Autodesk Fusion 360 part; units mm, degrees
sketch "Sketch1" plane through (0, 0, 0) normal (1, 0, 0) x (0, 1, 0)
  line L0 (180, 75) -> (-180, 75)
  line L1 (-240, 15) -> (-240, -75)
  line L2 (240, -75) -> (240, 15)
  line L3 (-240, -75) -> (-180, -75)
  line L4 (-180, -75) -> (-180, 75)
  line L5 (-240, 15) -> (-240, -75)
  line L6 (240, -75) -> (180, -75)
  line L7 (180, -75) -> (180, 75)
  line L8 (240, 15) -> (240, -75)
  line L9 (-180, 75) -> (180, 75)
  line L10 (240, 15) -> (-240, 15)
  line L11 (-240, 15) -> (-180, 75)
  line L12 (240, 15) -> (180, 75)
  line L13 (-240, -75) -> (-180, -75)
  line L14 (180, -75) -> (240, -75)
  line L15 (194.2857, 60.7143) -> (48, 15) construction
  line L16 (-194.2857, 60.7143) -> (-48, 15) construction
  line L17 (180, -56.25) -> (240, -75) construction
  line L18 (0, 55) -> (5, 55)
  line L19 (5, 35) -> (0, 35)
  line L20 (5, 65) -> (10, 65)
  line L21 (10, 65) -> (10, 25)
  line L22 (10, 25) -> (5, 25)
  line L23 (0, 75) -> (0, 55)
  line L24 (0, 35) -> (0, 15)
  line L25 (5, 25) -> (5, 35)
  line L26 (5, 55) -> (5, 65)
  dimension "d1" = 480
  dimension "d3" = 60
  dimension "d5" = 60
extrude "Extrude1" add sketch "Sketch1" along normal blind 3
sketch "Sketch2" plane through (0, 0, 0) normal (-1, 0, 0) x (0, -1, 0)
  line L0 (-180, -75) -> (-180, 15)
  line L1 (-180, 15) -> (180, 15)
  line L2 (180, 15) -> (180, -75)
  line L3 (180, -75) -> (240, -75)
  line L4 (240, -75) -> (240, 15)
  line L5 (240, 15) -> (180, 75)
  line L6 (180, 75) -> (-180, 75)
  line L7 (-180, 75) -> (-240, 15)
  line L8 (-240, 15) -> (-240, -75)
  line L9 (-240, -75) -> (-180, -75)
  line L10 (0, 55) -> (5, 55)
  line L11 (5, 35) -> (0, 35)
  line L12 (5, 65) -> (10, 65)
  line L13 (10, 65) -> (10, 25)
  line L14 (10, 25) -> (5, 25)
  line L15 (5, 25) -> (5, 35)
  line L16 (5, 55) -> (5, 65)
  line L17 (0, 55) -> (0, 75)
  line L18 (0, 35) -> (0, 15)
fillet "Fillet1" radius 25 2 edges at (1.5, -180, 15) (1.5, 180, 15)
fillet "Fillet2" radius 25 4 edges at (1.5, -240, 15) (1.5, -180, 75) (1.5, 180, 75) (1.5, 240, 15)
sketch "Sketch3" plane through (3, 0, 0) normal (1, 0, 0) x (0, 1, 0)
  arc A0 (240, 4.6447) -> (232.6777, 22.3223) centre (215, 4.6447) ccw
  line L0 (232.6777, 22.3223) -> (187.3223, 67.6777)
  arc A1 (187.3223, 67.6777) -> (169.6447, 75) centre (169.6447, 50) ccw
  line L1 (169.6447, 75) -> (-169.6447, 75)
  arc A2 (-169.6447, 75) -> (-187.3223, 67.6777) centre (-169.6447, 50) ccw
  line L2 (-187.3223, 67.6777) -> (-232.6777, 22.3223)
  arc A3 (-232.6777, 22.3223) -> (-240, 4.6447) centre (-215, 4.6447) ccw
  line L3 (-240, 4.6447) -> (-240, -75)
  line L4 (-240, -75) -> (-180, -75)
  line L5 (-180, -75) -> (-180, -10)
  arc A4 (-155, 15) -> (-180, -10) centre (-155, -10) ccw
  line L6 (-155, 15) -> (155, 15)
  arc A5 (180, -10) -> (155, 15) centre (155, -10) ccw
  line L7 (180, -10) -> (180, -75)
  line L8 (180, -75) -> (240, -75)
  line L9 (240, -75) -> (240, 4.6447)
The listing builds one solid part. Answer for the finished solid, in the listing's coordinates (mm). A direction names the side the tool comes from. Give positions to 0.01 mm unless a question says otherwise; leave off trailing zeros. Write each loop counter-clockwise with the first axis right and the second up, starting at its lowest first coordinate (ties: lowest second). Pieces come first, ordered by that corner, then holes.
Item 1: Which of the six approach directions +Z, -Z, +X, -X, +Y, -Y give full straight-line access (tool end or side, diameter ignored) to faces 1 (the cylindrical face through (1.521, 172.871, 7.482)), 2 (the flat face through (1, 210, 45))?
Item 2: Section C-C, the plane y = 67 is taken. Write down the section's boundary in (x, z), plus the area to 3 significant figures.
Item 3: Section A-A, the plane z = -25 is taken. Write down the section's boundary in (x, y), plus the area to 3 significant figures.
Item 4: Section D-D, the plane y = -161.5 is taken. Write down the section's boundary in (x, z), plus the area to 3 significant figures.
Item 5: Section B-B, the plane x = 0.5 is taken. Write down the section's boundary in (y, z), plus the area to 3 significant figures.
Item 6: Find the intervals of material crossed by line 1 along Y through (x, z) = (1.9, -59); line 2 along Z through (x, y) = (1.7, 33); line 3 along Z through (x, y) = (2.85, -209.5), in increasing order.
Completed:
1. face 1: -Z, +X, -X
1. face 2: +Z, +X, -X, +Y
2. outline: (0, 15) - (3, 15) - (3, 75) - (0, 75) - close
2. area: 180 mm2
3. outline: (0, -240) - (3, -240) - (3, -180) - (0, -180) - close; (0, 180) - (3, 180) - (3, 240) - (0, 240) - close
3. area: 360 mm2
4. outline: (0, 14.14) - (3, 14.14) - (3, 75) - (0, 75) - close
4. area: 183 mm2
5. outline: (-240, -75) - (-180, -75) - (-180, -10) arc R25 cw to (-155, 15) - (155, 15) arc R25 cw to (180, -10) - (180, -75) - (240, -75) - (240, 4.64) arc R25 ccw to (232.68, 22.32) - (187.32, 67.68) arc R25 ccw to (169.64, 75) - (-169.64, 75) arc R25 ccw to (-187.32, 67.68) - (-232.68, 22.32) arc R25 ccw to (-240, 4.64) - close
5. area: 36,200 mm2
6. line 1: y = -240 to -180, 180 to 240
6. line 2: z = 15 to 75
6. line 3: z = -75 to 45.5
